Here's how the part is built. I have some questions about the finished solid (model axes, mm). Round coordinates to 2 decimals unless told otherwise and drop trailing zeros. Order: outer loops, then holes, each group sorted by start corner. A loop starts at its lowest first (then second) coordinate and runs counter-clockwise, first axis right, second up. Notation, with made-up numbers: (-30.5, 12.25) -> (-11.5, 12.25) arc R35 ccw to (-11.5, 46.25) -> close; hole circle Ø10 at (84.25, -3). An arc over 180 degrees is marked (long way). Use a Markdown table: item, result. Add a question column.
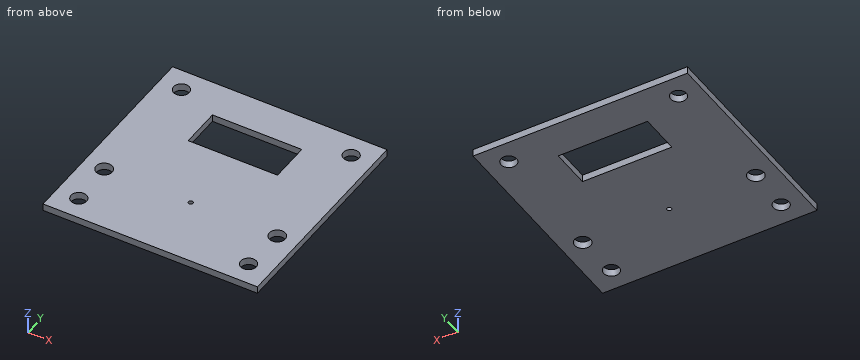
from build123d import *

# Parameters (mm, degrees)
F0_W     = 48
F0_H     = 1.6
F1_DEPTH = 48
F2_R     = 1.75
F2_R_2   = 1.8
F2_R_3   = 0.5
F3_DEPTH = 1.601
F4_W     = 20
F4_H     = 9
F5_DEPTH = 1.601
F6_W     = 48
F6_H     = 48
F6_R     = 1.75
F6_W_2   = 20
F6_H_2   = 9
F7_DEPTH = 5


with BuildPart() as f1:
    # F0 (on Right) → F1 (new body)
    with BuildSketch(Plane.YZ):
        Rectangle(F0_W, F0_H)
    extrude(amount=-F1_DEPTH)

    # F2 (on face) → F3 (cut, through all)
    with BuildSketch(Plane.XY.offset(0.8)):
        with Locations((-43, -19)):
            Circle(F2_R)
        with Locations((-43, 19)):
            Circle(F2_R)
        with Locations((-43.38, -9)):
            Circle(F2_R_2)
        with Locations((-4.62, -9)):
            Circle(F2_R_2)
        with Locations((-5, 19)):
            Circle(F2_R)
        with Locations((-5, -19)):
            Circle(F2_R)
        with Locations((-24, -9)):
            Circle(F2_R_3)
    extrude(amount=-F3_DEPTH, mode=Mode.SUBTRACT)

    # F4 (on face) → F5 (cut, through all)
    with BuildSketch(Plane.XY.offset(0.8)):
        with Locations((-24, 11.104)):
            Rectangle(F4_W, F4_H)
    extrude(amount=-F5_DEPTH, mode=Mode.SUBTRACT)


with BuildPart() as f7:
    # F6 (on Top) → F7 (new body)
    with BuildSketch(Plane.XY):
        Rectangle(F6_W, F6_H)
        with Locations((-19, -19)):
            Circle(F6_R, mode=Mode.SUBTRACT)
        with Locations((19, -19)):
            Circle(F6_R, mode=Mode.SUBTRACT)
        with Locations((-19, 19)):
            Circle(F6_R, mode=Mode.SUBTRACT)
        with Locations((0, 14.5)):
            Rectangle(F6_W_2, F6_H_2, mode=Mode.SUBTRACT)
        with Locations((19, 19)):
            Circle(F6_R, mode=Mode.SUBTRACT)
    extrude(amount=F7_DEPTH)


solid = f1.part
(1) I want a section at B-B on y = 11.5. List the corners of the cut face in (x, z) for me, and give its area (3 significant figures).
(2) I want a section at A-A on y = 19. List the corners of the cut face in (x, z) for me, and give its area (3 significant figures).
(3) I'm going to push a flat-ended pin straight in: P1, Ø4.5, axis at x = -5, y = 19, coming from the +Z side. Where does the tip first touch, or does it pass through?
(4) Please list where these lines run through material, in increasing order: probe 1 along Y at (x, z) = (-24, -0.25); probe 2 along Y at (x, z) = (-43, 0.4); probe 3 along Y at (x, z) = (-6, -0.05). Write a range as from..to.
(5) I want a section at D-D on x = -5. List the corners of the cut face in (y, z) for me, and give its area (3 significant figures).
(6) I want a section at C-C on z = 0.1. State how many separate pieces and enclosed holes the cut face has, and give its area (3 significant figures).
Output:
| question | item | result |
|---|---|---|
| 1 | outline | (-48, -0.8) -> (-34, -0.8) -> (-34, 0.8) -> (-48, 0.8) -> close; (-14, -0.8) -> (0, -0.8) -> (0, 0.8) -> (-14, 0.8) -> close |
| 1 | area | 44.8 mm² |
| 2 | outline | (-48, -0.8) -> (-44.75, -0.8) -> (-44.75, 0.8) -> (-48, 0.8) -> close; (-41.25, -0.8) -> (-6.75, -0.8) -> (-6.75, 0.8) -> (-41.25, 0.8) -> close; (-3.25, -0.8) -> (0, -0.8) -> (0, 0.8) -> (-3.25, 0.8) -> close |
| 2 | area | 65.6 mm² |
| 3 | P1 | z = 0.8 |
| 4 | probe 1 | -24..-9.5, -8.5..6.6, 15.6..24 |
| 4 | probe 2 | -24..-20.75, -17.25..-10.76, -7.24..17.25, 20.75..24 |
| 4 | probe 3 | -24..-20.44, -17.56..-10.16, -7.84..17.56, 20.44..24 |
| 5 | outline | (-24, -0.8) -> (-20.75, -0.8) -> (-20.75, 0.8) -> (-24, 0.8) -> close; (-17.25, -0.8) -> (-10.76, -0.8) -> (-10.76, 0.8) -> (-17.25, 0.8) -> close; (-7.24, -0.8) -> (17.25, -0.8) -> (17.25, 0.8) -> (-7.24, 0.8) -> close; (20.75, -0.8) -> (24, -0.8) -> (24, 0.8) -> (20.75, 0.8) -> close |
| 5 | area | 60.0 mm² |
| 6 | separate pieces | 1 |
| 6 | enclosed holes | 8 |
| 6 | area | 2,060 mm² |
